Drawing for the job (mm, zero at the part's lowest x, y, z). A direction names the side the tool comes from. Round coordinates to 2 decimals unless told otherwise and drop trailing zeros. Loops run counter-clockwise (first coordinate to the right, second up) from the corner with the lowest first, then second, coordinate; pieces in that order, holes last. Notation, with made-up numbers: (-27.5, 40.5) - (28.5, 40.5) arc R15 cw to (28.5, 53.5) - close; hole circle Ø6 at (68.25, 41). An arc over 180 degrees is marked (long way). Put each result on its own line as item: value.
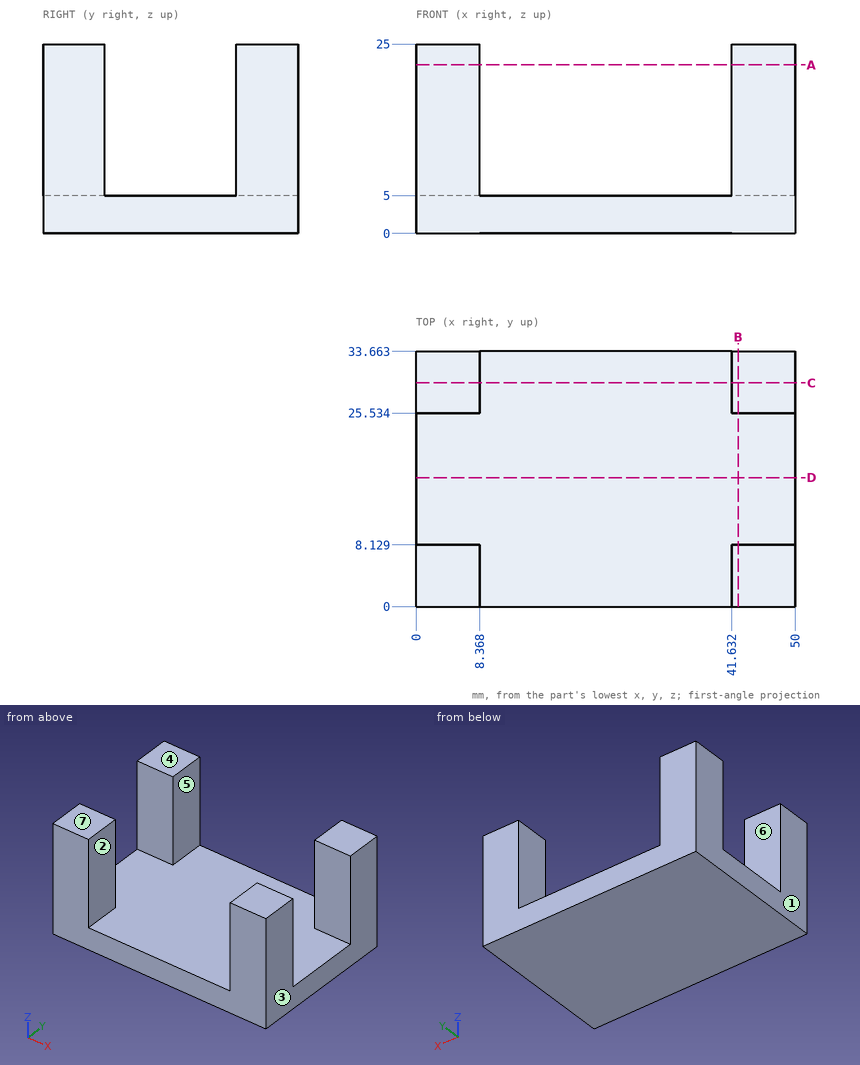
1. Band-saw the part on C-C (y = 29.5). List the corners of the cut face in (x, z).
A:
outline: (0, 0) - (50, 0) - (50, 25) - (41.63, 25) - (41.63, 5) - (8.37, 5) - (8.37, 25) - (0, 25) - close
2. Probe line 1 along X through (y, z) = (8, 18.25); line 2 along Z through (x, y) = (5, 18); line 3 along Y through (x, z) = (8, 10.5) (1 decimal). List the from-to ranges inside material, lowest first. Write a range as [from, to].
A:
line 1: x = [0, 8.37], [41.63, 50]
line 2: z = [0, 5]
line 3: y = [0, 8.1], [25.5, 33.7]
3. Band-saw the part on B-B (x = 42.5). List the corners of the cut face in (y, z) (1 decimal).
A:
outline: (0, 0) - (33.7, 0) - (33.7, 25) - (25.5, 25) - (25.5, 5) - (8.1, 5) - (8.1, 25) - (0, 25) - close
4. Band-saw the part on D-D (y = 17). List the corners of the cut face in (x, z).
A:
outline: (0, 0) - (50, 0) - (50, 5) - (0, 5) - close
5. Pin check, flat tips, straight feed: P1, Ø2.5, axis at y = 29.5, z = 17.5, coming from the -X side; P2, Ø4, axis at x = 15, y = 23.5, coming from the +Z side; P3, Ø8, axis at y = 14, z = 18.5, coming from the -X side. Stop position of each tip, or through.
A:
P1: stops at x = 0
P2: stops at z = 5
P3: passes through
6. Tool access for the marked faces 5, 6 and 7: list every direction of +Z, -Z, +X, -X, +Y, -Y with a clear straight run to the whole face (end or side of a thin tool).
A:
face 5: +Z, +Y, -Y
face 6: +Z, +X, -X
face 7: +Z, +X, -X, +Y, -Y
7. Two-plate mould, pull along X, no slides. Class the marked faces 1, 2, 3 and 4: pulls with the +X half, pulls with the -X half, needs draft (parallel to the pull), parting line crosses it, or undercut.
A:
face 1: pulls with the -X half
face 2: undercut
face 3: pulls with the +X half
face 4: needs draft
8. Band-saw the part on A-A (z = 22.25). List the corners of the cut face in (x, y) (1 decimal), plus the area to 3 significant figures.
A:
outline: (0, 0) - (8.4, 0) - (8.4, 8.1) - (0, 8.1) - close; (0, 25.5) - (8.4, 25.5) - (8.4, 33.7) - (0, 33.7) - close; (41.6, 0) - (50, 0) - (50, 8.1) - (41.6, 8.1) - close; (41.6, 25.5) - (50, 25.5) - (50, 33.7) - (41.6, 33.7) - close
area: 272 mm²
